from build123d import *

# Parameters (mm, degrees)
F1_DEPTH   = 0.8
F2_R       = 2
F3_DEPTH   = 15
F4_SIZE2   = 14.99999
F4_SIZE    = 1.99999
F4_2_SIZE2 = 14.99999
F4_2_SIZE  = 1.99999
F4_3_SIZE2 = 14.99999
F4_3_SIZE  = 1.99999
F4_4_SIZE2 = 14.99999
F4_4_SIZE  = 1.99999
F4_5_SIZE2 = 14.99999
F4_5_SIZE  = 1.99999
F4_6_SIZE2 = 14.99999
F4_6_SIZE  = 1.99999
F4_7_SIZE2 = 14.99999
F4_7_SIZE  = 1.99999
F4_8_SIZE2 = 14.99999
F4_8_SIZE  = 1.99999
F4_9_SIZE2 = 14.99999
F4_9_SIZE  = 1.99999


# Not quite as in the source:
# - a fillet or chamfer is up to 0.001 mm smaller than in the source, because OpenCascade refuses the exact size


with BuildPart() as f1:
    # F0 (on Top) → F1 (new body)
    with BuildSketch(Plane.XY):
        with BuildLine():
            ThreePointArc((-12.5, -7.5), (-11.0355339059, -11.0355339059), (-7.5, -12.5))
            Line((-7.5, -12.5), (7.5, -12.5))
            ThreePointArc((7.5, -12.5), (11.0355339059, -11.0355339059), (12.5, -7.5))
            Line((12.5, -7.5), (12.5, 7.5))
            ThreePointArc((12.5, 7.5), (11.0355339059, 11.0355339059), (7.5, 12.5))
            Line((7.5, 12.5), (-7.5, 12.5))
            ThreePointArc((-7.5, 12.5), (-11.0355339059, 11.0355339059), (-12.5, 7.5))
            Line((-12.5, 7.5), (-12.5, -7.5))
        make_face()
    extrude(amount=F1_DEPTH)

    # F2 (on face) → F3 (join)
    with BuildSketch(Plane.XY.offset(0.8)):
        with Locations((-8.5, -8.5)):
            Circle(F2_R)
        with Locations((-8.5, 0)):
            Circle(F2_R)
        with Locations((-8.5, 8.5)):
            Circle(F2_R)
        with Locations((0, -8.5)):
            Circle(F2_R)
        Circle(F2_R)
        with Locations((0, 8.5)):
            Circle(F2_R)
        with Locations((8.5, -8.5)):
            Circle(F2_R)
        with Locations((8.5, 0)):
            Circle(F2_R)
        with Locations((8.5, 8.5)):
            Circle(F2_R)
    extrude(amount=F3_DEPTH)

    # F4 (size 2 and 15 in the source; OpenCascade refuses exactly that, so slightly less here)
    f4_edges = [f1.edges().sort_by_distance(p)[0] for p in [
        (-10.5, -8.5, 15.8),
    ]]
    f4_side = f1.faces().sort_by_distance((-8.5, -8.5, 15.8))[0]
    chamfer(f4_edges, length=F4_SIZE, length2=F4_SIZE2, reference=f4_side)

    # F4#2 (size 2 and 15 in the source; OpenCascade refuses exactly that, so slightly less here)
    f4_2_edges = [f1.edges().sort_by_distance(p)[0] for p in [
        (-10.5, 0, 15.8),
    ]]
    f4_2_side = f1.faces().sort_by_distance((-8.5, 0, 15.8))[0]
    chamfer(f4_2_edges, length=F4_2_SIZE, length2=F4_2_SIZE2, reference=f4_2_side)

    # F4#3 (size 2 and 15 in the source; OpenCascade refuses exactly that, so slightly less here)
    f4_3_edges = [f1.edges().sort_by_distance(p)[0] for p in [
        (-10.5, 8.5, 15.8),
    ]]
    f4_3_side = f1.faces().sort_by_distance((-8.5, 8.5, 15.8))[0]
    chamfer(f4_3_edges, length=F4_3_SIZE, length2=F4_3_SIZE2, reference=f4_3_side)

    # F4#4 (size 2 and 15 in the source; OpenCascade refuses exactly that, so slightly less here)
    f4_4_edges = [f1.edges().sort_by_distance(p)[0] for p in [
        (-2, 8.5, 15.8),
    ]]
    f4_4_side = f1.faces().sort_by_distance((0, 8.5, 15.8))[0]
    chamfer(f4_4_edges, length=F4_4_SIZE, length2=F4_4_SIZE2, reference=f4_4_side)

    # F4#5 (size 2 and 15 in the source; OpenCascade refuses exactly that, so slightly less here)
    f4_5_edges = [f1.edges().sort_by_distance(p)[0] for p in [
        (-2, 0, 15.8),
    ]]
    f4_5_side = f1.faces().sort_by_distance((0, 0, 15.8))[0]
    chamfer(f4_5_edges, length=F4_5_SIZE, length2=F4_5_SIZE2, reference=f4_5_side)

    # F4#6 (size 2 and 15 in the source; OpenCascade refuses exactly that, so slightly less here)
    f4_6_edges = [f1.edges().sort_by_distance(p)[0] for p in [
        (-2, -8.5, 15.8),
    ]]
    f4_6_side = f1.faces().sort_by_distance((0, -8.5, 15.8))[0]
    chamfer(f4_6_edges, length=F4_6_SIZE, length2=F4_6_SIZE2, reference=f4_6_side)

    # F4#7 (size 2 and 15 in the source; OpenCascade refuses exactly that, so slightly less here)
    f4_7_edges = [f1.edges().sort_by_distance(p)[0] for p in [
        (6.5, -8.5, 15.8),
    ]]
    f4_7_side = f1.faces().sort_by_distance((8.5, -8.5, 15.8))[0]
    chamfer(f4_7_edges, length=F4_7_SIZE, length2=F4_7_SIZE2, reference=f4_7_side)

    # F4#8 (size 2 and 15 in the source; OpenCascade refuses exactly that, so slightly less here)
    f4_8_edges = [f1.edges().sort_by_distance(p)[0] for p in [
        (6.5, 0, 15.8),
    ]]
    f4_8_side = f1.faces().sort_by_distance((8.5, 0, 15.8))[0]
    chamfer(f4_8_edges, length=F4_8_SIZE, length2=F4_8_SIZE2, reference=f4_8_side)

    # F4#9 (size 2 and 15 in the source; OpenCascade refuses exactly that, so slightly less here)
    f4_9_edges = [f1.edges().sort_by_distance(p)[0] for p in [
        (6.5, 8.5, 15.8),
    ]]
    f4_9_side = f1.faces().sort_by_distance((8.5, 8.5, 15.8))[0]
    chamfer(f4_9_edges, length=F4_9_SIZE, length2=F4_9_SIZE2, reference=f4_9_side)


solid = f1.part
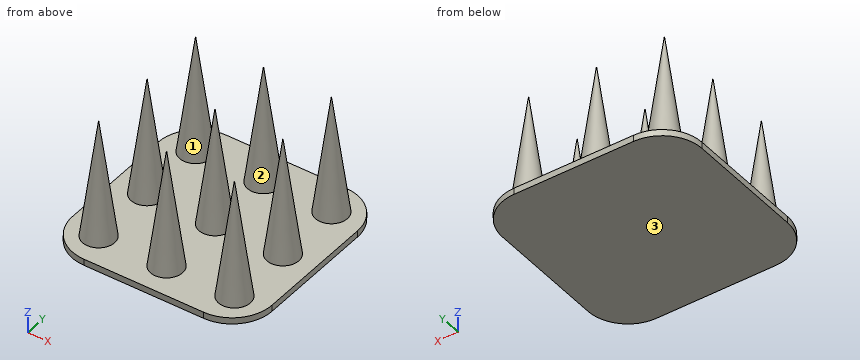
Design review of the part built by this model. Coordinates are the model's own, in mm. Face numbers are marked on the shaded views. Round coordinates to 2 decimals unless told otherwise and drop trailing zeros. Write each loop counter-clockwise with the first axis right and the second up, starting at its lowest first coordinate (ties: lowest second). Pieces come first, ordered by that corner, then holes. Notation, with made-up numbers: (62.25, 60.25) - (112.25, 60.25) arc R13 cw to (112.25, 80.25) - close; hole circle Ø6 at (41, 74). An arc over 180 degrees is marked (long way). Return JSON: item names as keys, results as strings. Group by question number.
Item 1: The part is to be moulded in two halves that separate along X. For the marked faces 1, 2 and 3, say which applies: pulls with the +X half, pulls with the -X half, needs draft (parallel to the pull), parting line crosses it, or undercut.
Item 2: We need section A-A on z = 5.75. Give the number of separate pieces and of enclosed holes in the cut face, and give its area (3 significant figures).
Item 3: We need section C-C on y = -3. Write out the cut boundary in (x, z), and give its area (3 significant figures).
Item 4: For probe 1 along X at (y, z) = (-0.5, 4.5); probe 2 along X at (y, z) = (-1.25, 1); probe 3 along Y at (x, z) = (-7, 3), list the stretches that pass through material, from the lowest coordinate up. Write a range as [from, to].
Item 5: Insertion check: P1, Ø8, axis at x = 1, z = 7, coming from the -Y side; P2, Ø8, axis at x = 8.5, y = -1, coming from the -Z side; P3, Ø2, axis at y = 9.5, z = 5.5, coming from the +X side; P4, Ø5, axis at y = -6.5, z = 9.5, coming from the -X side. Each pin has a flat end and moves straight along its axis. Give the tip position at first contact, or say it passes through.
Model answer:
{
 "1": {"face 1": "undercut", "face 2": "undercut", "face 3": "needs draft"},
 "2": {"separate pieces": "9", "enclosed holes": "0", "area": "50.8 mm²"},
 "3": {"outline": "(-12.5, 0) - (12.5, 0) - (12.5, 0.8) - (-12.5, 0.8) - close", "area": "20.0 mm²"},
 "4": {"probe 1": "x = [-9.92, -7.08], [-1.42, 1.42], [7.08, 9.92]", "probe 2": "x = [-10.03, -6.97], [-1.53, 1.53], [6.97, 10.03]", "probe 3": "y = [-9.31, -7.69], [-0.81, 0.81], [7.69, 9.31]"},
 "5": {"P1": "stops at y = -10.19", "P2": "stops at z = 0", "P3": "stops at x = 9.94", "P4": "stops at x = -9.55"}
}
